Study the drawing (mm; zero at the part's minimum x, y, z) and answer. A direction names the side the tool comes from. Coordinates: 2 decimals unless noted, no trailing zeros. Order: outer loops, then holes, each group sorted by start corner. A loop starts at its lowest first (then second) coordinate and runs counter-clockwise, first axis right, second up. Notation, with made-up numbers: M 34.25,61 L 73.25,61 A28 ccw 73.25,82 Z; hole C 7.25,10.5 d3. An arc over 180 degrees is marked long. Use a Markdown table: item, result. Add a question column.
1) Find the intervals of material crossed by probe 1 along Y at (x, z) = (14, 8.5); probe 2 along X at (y, z) = (16.25, 8); probe 3 along X at (y, z) = (3.75, 11.75), in increasing order. Write a range as [from, to].
2) The mould has two halves that part along X. Classify the marked faces 1, 2, 3 and 4: released by +X, released by -X, zero draft, split by the parting line, or undercut.
3) For the marked faces 5 and 6, determine the directions among +Z, -Z, +X, -X, +Y, -Y from which every point of the face is accessible in a straight line to the end or side of a thin tool.
4) Find section A-A on x = 8. Write down the section's boundary in (y, z).
5) Find section B-B on z = 8. Write down the section's boundary in (x, y).
6) Each of these flat-tipped pins is pushed along its axis until it touches: pin 1 Ø6 at (y, z) = (15.5, 12.5) entering from +X; pin 2 Ø1.5 at (x, y) = (2.5, 17) entering from -Z; pin 3 Ø2 at (y, z) = (7, 11) entering from +X. Where does it stop, or does it pass through?
7) Find section D-D on z = 1.25. Write down the section's boundary in (x, y).
8) Find section C-C on y = 3.5. Write down the section's boundary in (x, z).
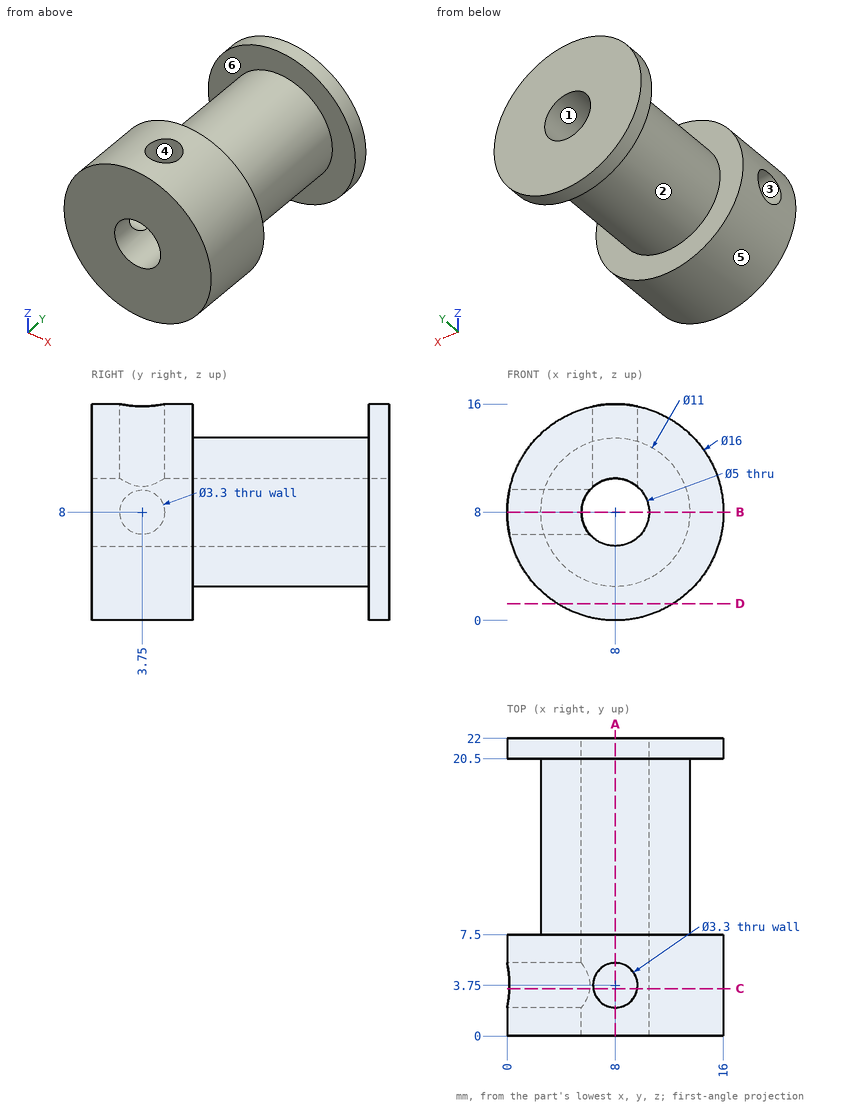
Check result:
| question | item | result |
|---|---|---|
| 1 | probe 1 | y = [0, 7.5], [20.5, 22] |
| 1 | probe 2 | x = [2.5, 5.5], [10.5, 13.5] |
| 1 | probe 3 | x = [0.93, 6.35], [9.65, 15.07] |
| 2 | face 1 | undercut |
| 2 | face 2 | split by the parting line |
| 2 | face 3 | zero draft |
| 2 | face 4 | undercut |
| 3 | face 5 | +Y, -Y |
| 3 | face 6 | none |
| 4 | outline | M 0,0 L 7.5,0 L 7.5,2.5 L 20.5,2.5 L 20.5,0 L 22,0 L 22,5.5 L 0,5.5 Z; M 0,10.5 L 2.1,10.5 L 2.1,16 L 0,16 Z; M 5.4,10.5 L 22,10.5 L 22,16 L 20.5,16 L 20.5,13.5 L 7.5,13.5 L 7.5,16 L 5.4,16 Z |
| 5 | outline | M 0,0 L 5.5,0 L 5.5,2.1 L 0,2.1 Z; M 0,5.4 L 5.5,5.4 L 5.5,22 L 0,22 L 0,20.5 L 2.5,20.5 L 2.5,7.5 L 0,7.5 Z; M 10.5,0 L 16,0 L 16,7.5 L 13.5,7.5 L 13.5,20.5 L 16,20.5 L 16,22 L 10.5,22 Z |
| 6 | pin 1 | stops at x = 13.29 |
| 6 | pin 2 | stops at z = 5.23 |
| 6 | pin 3 | stops at x = 15.75 |
| 7 | outline | M 3.71,0 L 12.29,0 L 12.29,7.5 L 3.71,7.5 Z; M 3.71,20.5 L 12.29,20.5 L 12.29,22 L 3.71,22 Z |
| 8 | outline | M 0.17,6.37 A8 ccw long 9.63,15.83 L 9.63,9.89 A2.5 cw long 6.11,6.37 Z; M 0.17,9.63 L 6.11,9.63 A2.5 cw 6.37,9.89 L 6.37,15.83 A8 ccw Z |
